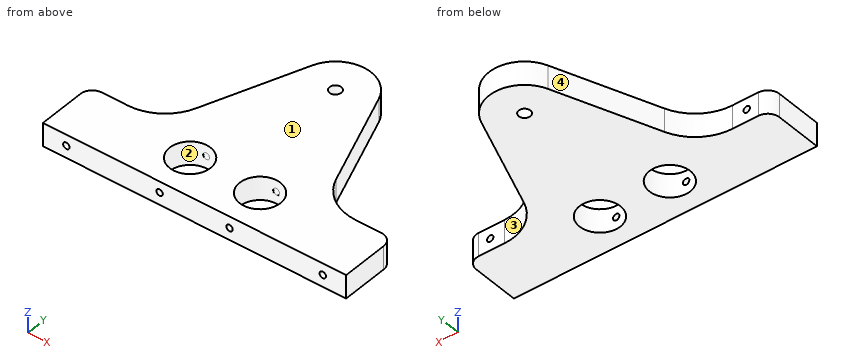
```python
from build123d import *

# Parameters (mm, degrees)
F0_R     = 17.5
F0_R_2   = 5
F1_DEPTH = 20
F2_R     = 2.75
F3_DEPTH = 50.001
F4_R     = 40
F5_R     = 10


with BuildPart() as f1:
    # F0 (on Top) → F1 (new body)
    with BuildSketch(Plane.XY):
        with BuildLine():
            Line((-130, 0), (130, 0))
            Line((130, 0), (130, 50))
            Line((130, 50), (70, 50))
            Line((70, 50), (28.564314, 160.69252))
            ThreePointArc((28.564314, 160.69252), (0, 180.5), (-28.564314, 160.69252))
            Line((-28.564314, 160.69252), (-70, 50))
            Line((-70, 50), (-130, 50))
            Line((-130, 50), (-130, 0))
        make_face()
        with Locations((-30, 32.5)):
            Circle(F0_R, mode=Mode.SUBTRACT)
        with Locations((30, 32.5)):
            Circle(F0_R, mode=Mode.SUBTRACT)
        with Locations((0, 150)):
            Circle(F0_R_2, mode=Mode.SUBTRACT)
    extrude(amount=F1_DEPTH)

    # F2 (on face) → F3 (cut, through all)
    with BuildSketch(Plane(origin=(0, 50, 0), x_dir=(-1, 0, 0), z_dir=(0, 1, 0))):
        with Locations((-110, 10.207103)):
            Circle(F2_R)
        with Locations((110, 10.485964)):
            Circle(F2_R)
        with Locations((-30, 10.207103)):
            Circle(F2_R)
        with Locations((30, 10.485964)):
            Circle(F2_R)
    extrude(amount=-F3_DEPTH, mode=Mode.SUBTRACT)

    # F4
    f4_edges = [f1.edges().sort_by_distance(p)[0] for p in [
        (70, 50, 10),
        (-70, 50, 10),
    ]]
    fillet(f4_edges, radius=F4_R)

    # F5
    f5_edges = [f1.edges().sort_by_distance(p)[0] for p in [
        (130, 50, 10),
        (-130, 50, 10),
    ]]
    fillet(f5_edges, radius=F5_R)


solid = f1.part
```
CAD build for the part. Positions are in the model's coordinates, mm. Face numbers are marked on the shaded views. Coordinates: 2 decimals unless noted, no trailing zeros. Order: outer loops, then holes, each group sorted by start corner. A loop starts at its lowest first (then second) coordinate and runs counter-clockwise, first axis right, second up. Notation, with made-up numbers: M 25,-16.75 L 30,-16.75 A37 ccw 30,20.25 Z; hole C 40,79.5 d7. An arc over 180 degrees is marked long. Answer as CSV lines item,"result".
1) Drill centre lines: L1, parallel to X at y = 28, z = 19.25; L2, parallel to Z at x = 30, y = 7.5; L3, parallel to Y at x = 115, z = 9.75. Where is each one in solid material? Low to high. Write a range as from..to.
Verdict:
L1,"-130..-46.91, -13.09..13.09, 46.91..130"
L2,"0..7.46, 12.96..20"
L3,"0..50"
2) Cut at A-A (x = 0). List the corners of the cut face in (y, z), then the cut area to 3 significant figures.
Verdict:
outline,"M 0,0 L 145,0 L 145,20 L 0,20 Z; M 155,0 L 180.5,0 L 180.5,20 L 155,20 Z"
area,"3,410 mm2"
3) Cut at B-B (z = 3.75). List the corners of the cut face in (x, y).
Verdict:
outline,"M -130,0 L 130,0 L 130,40 A10 ccw 120,50 L 97.74,50 A40 cw 60.28,75.98 L 28.56,160.69 A30.5 ccw -28.56,160.69 L -60.28,75.98 A40 cw -97.74,50 L -120,50 A10 ccw -130,40 Z; hole C -30,32.5 d35; hole C 0,150 d10; hole C 30,32.5 d35"
4) Mould opens along X. For the marked faces 1, 2, 3 and 4 say: released by +X, released by -X, zero draft, split by the parting line, or undercut.
Verdict:
face 1,"zero draft"
face 2,"undercut"
face 3,"released by +X"
face 4,"released by -X"
5) Cut at D-D (y = 150). List the corners of the cut face in (x, z), then the cut area to 3 significant figures.
Verdict:
outline,"M -32.57,0 L -5,0 L -5,20 L -32.57,20 Z; M 5,0 L 32.57,0 L 32.57,20 L 5,20 Z"
area,"1,100 mm2"
6) Cut at C-C (y = 32.5). List the corners of the cut face in (x, z), then the cut area to 3 significant figures.
Verdict:
outline,"M -130,0 L -47.5,0 L -47.5,20 L -130,20 Z; M -12.5,0 L 12.5,0 L 12.5,20 L -12.5,20 Z; M 47.5,0 L 130,0 L 130,20 L 47.5,20 Z; hole C -110,10.49 d5.5; hole C 110,10.21 d5.5"
area,"3,750 mm2"
7) Flat gauge pins, fed straight in: P1, Ø4.5, axis at x = -110, z = 10.49, coming from the +Y side; P2, Ø10, axis at y = 74, z = 3.5, coming from the +X side; P3, Ø1.5, axis at y = 113, z = 7, coming from the +X side; P4, Ø10, axis at x = 112.5, z = 9, coming from the +Y side. Where does each tip first touch, or does it go through?
Verdict:
P1,"through"
P2,"x = 63.69"
P3,"x = 46.7"
P4,"y = 50"
